```python
from build123d import *

# Parameters (mm, degrees)
F0_R      = 5.85
F1_DEPTH  = 25
F1_TAPER  = 3
F2_DEPTH  = 25
F2_FACE_R = 4.5398055179
F3_DEPTH  = 25
F3_TAPER  = -3
F3_FACE_R = 5.85
F4_DEPTH  = 20
F4_TAPER  = 10
F5_W      = 1
F5_H      = 1
F6_DEPTH  = 20


with BuildPart() as f1:
    # F0 (on Top) → F1 (new body)
    with BuildSketch(Plane.XY):
        Circle(F0_R)
    extrude(amount=F1_DEPTH, taper=F1_TAPER)

    # F2 (add): a face of the model
    f2_faces = [f1.faces().sort_by_distance(p)[0] for p in [
        (0, 0, 25),
    ]]
    extrude(f2_faces, amount=F2_DEPTH)

    # F2_face (on face) → F3 (join)
    with BuildSketch(Plane.XY.offset(50)):
        Circle(F2_FACE_R)
    extrude(amount=F3_DEPTH, taper=F3_TAPER)

    # F3_face (on face) → F4 (join)
    with BuildSketch(Plane.XY.offset(75)):
        Circle(F3_FACE_R)
    extrude(amount=F4_DEPTH, taper=F4_TAPER)

    # F5 (on face) → F6 (cut)
    with BuildSketch(Plane.XY.offset(95)):
        with BuildLine():
            Line((-0.5, 2.2690236148), (-0.5, 0.5))
            Line((-0.5, 0.5), (0.5, 0.5))
            Line((0.5, 0.5), (0.5, 2.2690236148))
            ThreePointArc((0.5, 2.2690236148), (0, 2.3234603858), (-0.5, 2.2690236148))
        make_face()
        with BuildLine():
            ThreePointArc((-2.2690236148, 0.5), (-2.3234603858, 0), (-2.2690236148, -0.5))
            Line((-2.2690236148, -0.5), (-0.5, -0.5))
            Line((-0.5, -0.5), (-0.5, 0.5))
            Line((-0.5, 0.5), (-2.2690236148, 0.5))
        make_face()
        with BuildLine():
            Line((0.5, -0.5), (-0.5, -0.5))
            Line((-0.5, -0.5), (-0.5, -2.2690236148))
            ThreePointArc((-0.5, -2.2690236148), (0, -2.3234603858), (0.5, -2.2690236148))
            Line((0.5, -2.2690236148), (0.5, -0.5))
        make_face()
        with BuildLine():
            Line((0.5, 0.5), (0.5, -0.5))
            Line((0.5, -0.5), (2.2690236148, -0.5))
            ThreePointArc((2.2690236148, -0.5), (2.3098111014, -0.2514773161), (2.3234603858, 0))
            ThreePointArc((2.3234603858, 0), (2.3098111014, 0.2514773161), (2.2690236148, 0.5))
            Line((2.2690236148, 0.5), (0.5, 0.5))
        make_face()
        Rectangle(F5_W, F5_H)
        with BuildLine():
            Line((-10.1169492777, 0.5), (-10.1169492777, -0.5))
            Line((-10.1169492777, -0.5), (-2.2690236148, -0.5))
            ThreePointArc((-2.2690236148, -0.5), (-2.3234603858, 0), (-2.2690236148, 0.5))
            Line((-2.2690236148, 0.5), (-10.1169492777, 0.5))
        make_face()
        with BuildLine():
            ThreePointArc((0.5, -2.2690236148), (0, -2.3234603858), (-0.5, -2.2690236148))
            Line((-0.5, -2.2690236148), (-0.5, -11.6822896525))
            Line((-0.5, -11.6822896525), (0.5, -11.6822896525))
            Line((0.5, -11.6822896525), (0.5, -2.2690236148))
        make_face()
        with BuildLine():
            ThreePointArc((2.3234603858, 0), (2.3098111014, -0.2514773161), (2.2690236148, -0.5))
            Line((2.2690236148, -0.5), (10.1169492777, -0.5))
            Line((10.1169492777, -0.5), (10.1169492777, 0.5))
            Line((10.1169492777, 0.5), (2.2690236148, 0.5))
            ThreePointArc((2.2690236148, 0.5), (2.3098111014, 0.2514773161), (2.3234603858, 0))
        make_face()
        with BuildLine():
            Line((-0.5, 11.6822896525), (-0.5, 2.2690236148))
            ThreePointArc((-0.5, 2.2690236148), (0, 2.3234603858), (0.5, 2.2690236148))
            Line((0.5, 2.2690236148), (0.5, 11.6822896525))
            Line((0.5, 11.6822896525), (-0.5, 11.6822896525))
        make_face()
    extrude(amount=-F6_DEPTH, mode=Mode.SUBTRACT)


solid = f1.part
```
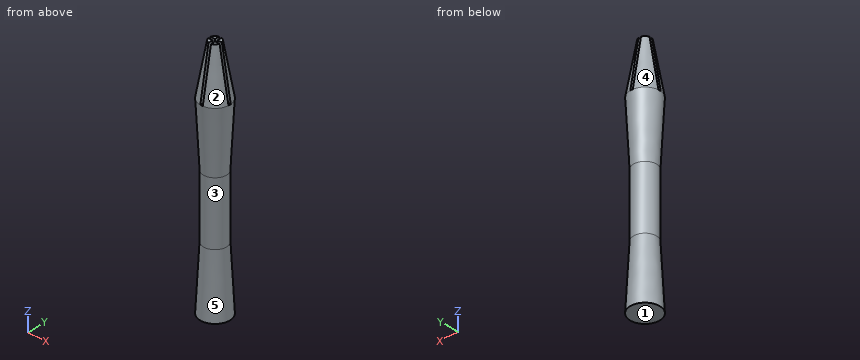
Could you check a few things on this model? Use its own coordinates, in mm. Face numbers are marked on the shaded views. A direction names the side the tool comes from. Give positions to 0.01 mm unless a question says otherwise; leave off trailing zeros. Loops run counter-clockwise (first coordinate to the right, second up) from the corner with the lowest first, then second, coordinate; pieces in that order, holes last. Notation, with made-up numbers: (-30, 5) -> (15, 5) arc R38 cw to (15, 43) -> close; hole circle Ø7 at (-9, 43.5). An arc over 180 degrees is marked (long way). Put each result on its own line as item: value.
(1) Please list where these lines run through material, in increasing order: probe 1 along Z at (x, y) = (4.5, -0.25); probe 2 along Y at (x, z) = (-1, 83); probe 3 along X at (y, z) = (-4, 51). Write a range as [from, to].
Computed:
probe 1: [0, 75]
probe 2: [-4.33, -0.5], [0.5, 4.33]
probe 3: [-2.26, 2.26]
(2) Imagine slicing it at C-C on z = 11. Write out the boundary of the cut face in (x, y), plus the area to 3 significant figures.
Computed:
outline: circle Ø10.55 at (0, 0)
area: 87.4 mm^2
(3) I'm going to push flat-ended pins straight in: pin 1 Ø4.5 at (x, z) = (-3, 89.5) entering from -Y; pin 2 Ø4.5 at (x, z) = (-3.5, 82.5) entering from +Y; pin 3 Ø6 at (y, z) = (3.5, 89.5) entering from +X. Where does each tip first touch, or does it pass through?
Computed:
pin 1: y = -3.33
pin 2: y = 4.46
pin 3: x = 3.44
(4) Imagine slicing it at B-B on z = 46. Write out the boundary of the cut face in (x, y), plus the area to 3 significant figures.
Computed:
outline: circle Ø9.08 at (0, 0)
area: 64.7 mm^2
(5) Thinking about a two-plate mould opening in Z: for the marked faces 1, 2 and 3, which applies, pulls with the +Z half, pulls with the -Z half, needs draft (parallel to the pull), parting line crosses it, or undercut?
Computed:
face 1: pulls with the -Z half
face 2: pulls with the +Z half
face 3: undercut
(6) For the marked faces 4 and 5, which set-ups out of +Z, -Z, +X, -X, +Y, -Y let a thin tool reach every point of the face, with its end or its side?
Computed:
face 4: +Z, -X, +Y
face 5: none
(7) Imagine slicing it at A-A on z = 85.5. Write out the boundary of the cut face in (x, y), plus the area to 3 significant figures.
Computed:
outline: (-3.97, -0.5) arc R4 ccw to (-0.5, -3.97) -> (-0.5, -0.5) -> close; (-3.97, 0.5) -> (-0.5, 0.5) -> (-0.5, 3.97) arc R4 ccw to start; (0.5, -3.97) arc R4 ccw to (3.97, -0.5) -> (0.5, -0.5) -> close; (0.5, 0.5) -> (3.97, 0.5) arc R4 ccw to (0.5, 3.97) -> close
area: 35.3 mm^2
